Design review of the part shown in the three views and the two pictorial views. Dimensions are in mm from the part's minimum x, y and z. A direction names the side the tool comes from. Round coordinates to 2 decimals unless told otherwise and drop trailing zeros. Write each loop counter-clockwise with the first axis right and the second up, starting at its lowest first coordinate (ties: lowest second). Pieces come first, ordered by that corner, then holes. Notation, with made-up numbers: (-24, 40) - (16, 40) arc R25 cw to (16, 77) - close; hole circle Ø11 at (-15, -25.75). An arc over 180 degrees is marked (long way). Use one line per item in the form item = value.
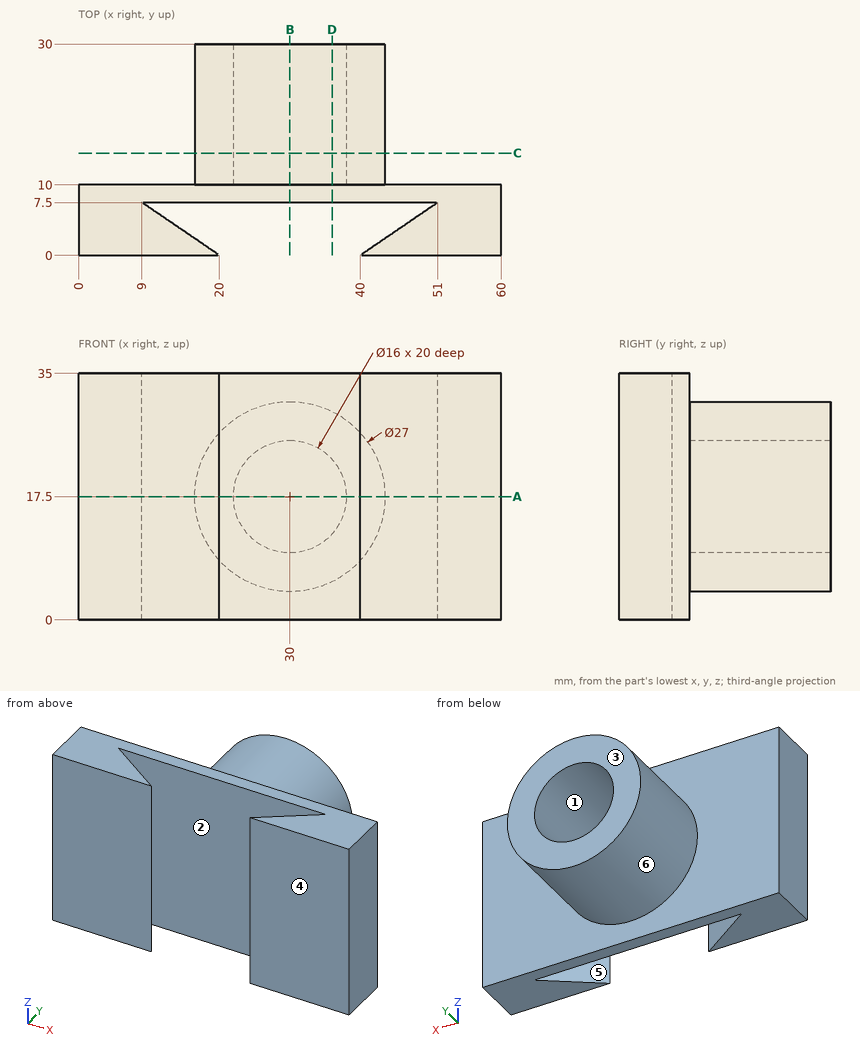
Q1. We need section A-A on z = 17.5. Write out the cut boundary in (x, y).
Calculated:
outline = (0, 0) - (20, 0) - (9, 7.5) - (51, 7.5) - (40, 0) - (60, 0) - (60, 10) - (43.5, 10) - (43.5, 30) - (38, 30) - (38, 10) - (22, 10) - (22, 30) - (16.5, 30) - (16.5, 10) - (0, 10) - close
Q2. For P1, Ø6, axis at x = 34, z = 4.5, coming from the -Y side; P2, Ø1.5, axis at y = 16.5, z = 20, coming from the +X side; P3, Ø5, axis at x = 21.5, y = 16.5, coming from the -Z side, all flat-tipped, find the tip position at first contact; note any pin that passes through.
Calculated:
P1 = 7.5
P2 = 43.39
P3 = 5.41
Q3. To check wall thickness, follow line 1 along X through (y, z) = (20, 17.5); line 2 along X through (y, z) = (2.75, 20.5); line 3 along Y through (x, z) = (53, 2). State the ranges of each line that lie inside material, in increasing order. Write a range as from..to.
Calculated:
line_1 = 16.5..22, 38..43.5
line_2 = 0..15.97, 44.03..60
line_3 = 0..10
Q4. We need section D-D on x = 36. Write out the cut boundary in (y, z).
Calculated:
outline = (7.5, 0) - (10, 0) - (10, 5.41) - (30, 5.41) - (30, 12.21) - (10, 12.21) - (10, 22.79) - (30, 22.79) - (30, 29.59) - (10, 29.59) - (10, 35) - (7.5, 35) - close
Q5. We need section C-C on y = 14.5. Write out the cut boundary in (x, z), then the cut area to 3 significant figures.
Calculated:
outline = circle Ø27 at (30, 17.5); hole circle Ø16 at (30, 17.5)
area = 371 mm2
Q6. Draft analysis for pull direction Y (two halves, no side actions). For the marked faces 4, 5 and 6, state which applies: released by +Y, released by -Y, zero draft, split by the parting line, or undercut.
Calculated:
face_4 = released by -Y
face_5 = undercut
face_6 = zero draft
Q7. We need section B-B on x = 30. Write out the cut boundary in (y, z).
Calculated:
outline = (7.5, 0) - (10, 0) - (10, 4) - (30, 4) - (30, 9.5) - (10, 9.5) - (10, 25.5) - (30, 25.5) - (30, 31) - (10, 31) - (10, 35) - (7.5, 35) - close
Q8. Machinability: for the marked faces 1, 2 and 3, which of the approach directions +Z, -Z, +X, -X, +Y, -Y give a long, thin tool a straight path to every point of the face, cutting with its end or side? Answer none if there is none.
Calculated:
face_1 = +Y
face_2 = +Z, -Z
face_3 = +Z, -Z, +X, -X, +Y
